from build123d import *

# Parameters (mm, degrees)
BASE_EXTRUDE_DEPTH = 101.6
HOLE1_START        = -18.034
HOLE1_OUTLINE_R    = 7.14375
HOLE1_DEPTH        = 2.6924
LPATTERN1_COUNT    = 2
LPATTERN1_PITCH    = 47.625


# Read off the part's stored shape, not the designer's step: Hole1
with BuildPart() as part:
    # Sketch1 → Base-Extrude (new body)
    with BuildSketch(Plane.XY):
        with BuildLine():
            Line((-20.6375, 18.4785), (-20.6375, -15.3416))
            ThreePointArc((-20.6375, -15.3416), (-19.848914298, -17.245414298), (-17.9451, -18.034))
            Line((-17.9451, -18.034), (17.9451, -18.034))
            ThreePointArc((17.9451, -18.034), (19.848914298, -17.245414298), (20.6375, -15.3416))
            Line((20.6375, -15.3416), (20.6375, 18.4785))
            ThreePointArc((20.6375, 18.4785), (15.875, 23.241), (11.1125, 18.4785))
            Line((11.1125, 18.4785), (11.1125, 17.44345))
            ThreePointArc((11.1125, 17.44345), (12.4587, 16.09725), (13.8049, 17.44345))
            Line((13.8049, 17.44345), (13.8049, 18.4785))
            ThreePointArc((13.8049, 18.4785), (15.875, 20.5486), (17.9451, 18.4785))
            Line((17.9451, 18.4785), (17.9451, -15.3416))
            Line((17.9451, -15.3416), (-17.9451, -15.3416))
            Line((-17.9451, -15.3416), (-17.9451, 18.4785))
            ThreePointArc((-17.9451, 18.4785), (-15.875, 20.5486), (-13.8049, 18.4785))
            Line((-13.8049, 18.4785), (-13.8049, 17.44345))
            ThreePointArc((-13.8049, 17.44345), (-12.4587, 16.09725), (-11.1125, 17.44345))
            Line((-11.1125, 17.44345), (-11.1125, 18.4785))
            ThreePointArc((-11.1125, 18.4785), (-15.875, 23.241), (-20.6375, 18.4785))
        make_face()
    extrude(amount=BASE_EXTRUDE_DEPTH)

    # Hole1 outline → Hole1 (cut)
    with BuildSketch(Plane(origin=(0, 0, 0), x_dir=(1, 0, 0), z_dir=(0, 1, 0)).offset(HOLE1_START)):
        with Locations((0, -23.8125)):
            Circle(HOLE1_OUTLINE_R)
    hole1 = extrude(amount=HOLE1_DEPTH, mode=Mode.SUBTRACT)

    # LPattern1: Hole1 ×2
    with Locations(*[(0, 0, i * LPATTERN1_PITCH) for i in range(1, LPATTERN1_COUNT)]):
        add(hole1, mode=Mode.SUBTRACT)


solid = part.part
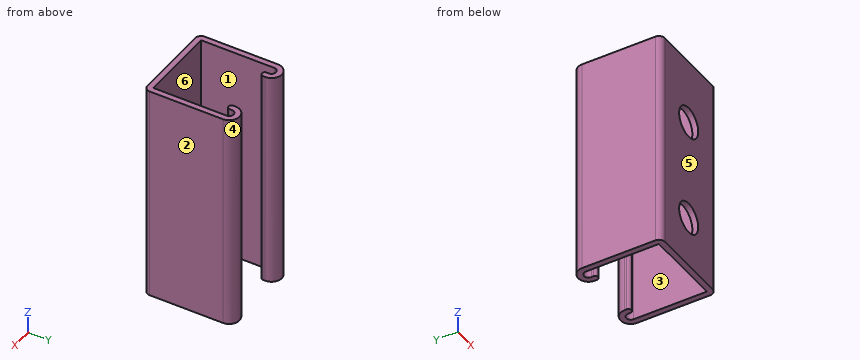
Check sheet for the modelled part. Datum: model origin and axes. Units: mm. Face numbers are marked on the shaded views. A direction names the side the tool comes from. Round coordinates to 2 decimals unless told otherwise and drop trailing zeros. Write each loop counter-clockwise with the first axis right and the second up, starting at its lowest first coordinate (ties: lowest second). Pieces come first, ordered by that corner, then holes. Notation, with made-up numbers: (72.5, 55.5) -> (87.5, 55.5) arc R30 ccw to (87.5, 83.5) -> close; hole circle Ø9 at (13.5, 70). An arc over 180 degrees is marked (long way). Answer as CSV lines item,"result". Start each with the question number.
1) Material ranges on line 1 (Z direction, x = 0, y = -16); line 2 (X direction, y = -4, z = 45); line 3 (Y direction, x = 1, z = 47.5), recorded low to high. Write a range as from..to.
2) Tool access check on the marked faces 1 and 2. Record the directions out of +Z, -Z, +X, -X, +Y, -Y that give a thin tool (end or side, any length) a straight path to the whole face; none if there is none.
3) Section check A-A on y = -2. Enter the section's corners in (x, z).
4) Section check D-D on z = 25.5. Enter the section's corners in (x, y) (1 decimal), and give its area (3 significant figures).
5) Section check B-B on x = 0. Enter the section's corners in (y, z), and give its area (3 significant figures).
6) Section check C-C on z = 9. Enter the section's corners in (x, y) (1 decimal).
7) Release check for a two-part mould opening along Y. For the marked faces 3, 4, 5 and 6 record: pulls with the +Y half, pulls with the -Y half, needs draft (parallel to the pull), parting line crosses it, or undercut.
8) Go/stop test with a flat-tipped pin: P1, Ø11, axis at x = -3.5, z = 63.5, coming from the +Y side. Record where the tip stops, or that it passes through.
Found:
1,line 1,"z = 0..16.67, 30.96..64.29, 78.58..101.6"
1,line 2,"x = -20.64..-17.95, 17.95..20.64"
1,line 3,"y = -18.03..-15.34"
2,face 1,"+Z, -Z"
2,face 2,"+Z, -Z, +X, +Y, -Y"
3,outline,"(-20.64, 0) -> (-17.95, 0) -> (-17.95, 101.6) -> (-20.64, 101.6) -> close; (17.95, 0) -> (20.64, 0) -> (20.64, 101.6) -> (17.95, 101.6) -> close"
4,outline,"(-20.6, -15.3) arc R2.7 ccw to (-17.9, -18) -> (-6.9, -18) -> (-6.9, -15.3) -> (-17.9, -15.3) -> (-17.9, 18.5) arc R2.1 cw to (-13.8, 18.5) -> (-13.8, 17.4) arc R1.3 ccw to (-11.1, 17.4) -> (-11.1, 18.5) arc R4.8 ccw to (-20.6, 18.5) -> close; (6.9, -18) -> (17.9, -18) arc R2.7 ccw to (20.6, -15.3) -> (20.6, 18.5) arc R4.8 ccw to (11.1, 18.5) -> (11.1, 17.4) arc R1.3 ccw to (13.8, 17.4) -> (13.8, 18.5) arc R2.1 cw to (17.9, 18.5) -> (17.9, -15.3) -> (6.9, -15.3) -> close"
4,area,"322 mm^2"
5,outline,"(-18.03, 0) -> (-15.34, 0) -> (-15.34, 16.67) -> (-18.03, 16.67) -> close; (-18.03, 30.96) -> (-15.34, 30.96) -> (-15.34, 64.29) -> (-18.03, 64.29) -> close; (-18.03, 78.58) -> (-15.34, 78.58) -> (-15.34, 101.6) -> (-18.03, 101.6) -> close"
5,area,"197 mm^2"
6,outline,"(-20.6, -15.3) arc R2.7 ccw to (-17.9, -18) -> (17.9, -18) arc R2.7 ccw to (20.6, -15.3) -> (20.6, 18.5) arc R4.8 ccw to (11.1, 18.5) -> (11.1, 17.4) arc R1.3 ccw to (13.8, 17.4) -> (13.8, 18.5) arc R2.1 cw to (17.9, 18.5) -> (17.9, -15.3) -> (-17.9, -15.3) -> (-17.9, 18.5) arc R2.1 cw to (-13.8, 18.5) -> (-13.8, 17.4) arc R1.3 ccw to (-11.1, 17.4) -> (-11.1, 18.5) arc R4.8 ccw to (-20.6, 18.5) -> close"
7,face 3,"undercut"
7,face 4,"pulls with the +Y half"
7,face 5,"pulls with the -Y half"
7,face 6,"undercut"
8,P1,"stops at y = -15.34"
